```python
from build123d import *

# Parameters (mm, degrees)
SKETCH1_R               = 152.4
BOSS_EXTRUDE1_DEPTH     = 19.05
SKETCH5_R               = 55
CUT_EXTRUDE1_DEPTH      = 217.366407975
F_3_8_CLEARANCE_HOLE1_D = 9.8044


with BuildPart() as part:
    # Sketch1 → Boss-Extrude1 (new body)
    with BuildSketch(Plane.XY):
        with Locations(Location((0, 0, 0), (0, 0, 180))):
            Circle(SKETCH1_R)
    extrude(amount=BOSS_EXTRUDE1_DEPTH)

    # Sketch5 → Cut-Extrude1 (cut, through all)
    with BuildSketch(Plane(origin=(0, 0, 0), x_dir=(-1, 0, 0), z_dir=(0, 0, -1))):
        Circle(SKETCH5_R)
    extrude(amount=-CUT_EXTRUDE1_DEPTH, mode=Mode.SUBTRACT)

    # 3/8 Clearance Hole1 (through all)
    with Locations(Plane.XY.offset(19.05)):
        with Locations((60.285109168, 24.861699689), (60.262270723, -25.040419345), (-24.942124319, -60.287558469), (-60.212101884, -24.985282473), (24.959994735, -60.310396903), (-60.212101884, 24.861699689), (-24.88698742, 60.186814133), (25.015131626, 60.163975676)):
            Hole(F_3_8_CLEARANCE_HOLE1_D / 2)


solid = part.part
```
Geometry check sheet. Reference: the model listing, model coordinates, mm. Coordinates: 2 decimals unless noted, no trailing zeros. Order: outer loops, then holes, each group sorted by start corner. A loop starts at its lowest first (then second) coordinate and runs counter-clockwise, first axis right, second up.
Q1. Draft check along X on faces 1 (the face through (-27.2, -64.64, 9.39)), 2 (the face through (33.037, 148.776, 9.392)), 3 (the face through (-66, -2, 0)). Enter one of: released by +X, released by -X, zero draft, split by the parting line, or undercut.
Reply:
face 1: undercut
face 2: split by the parting line
face 3: zero draft
Q2. Sectioned sample at C-C on z = 6.75. Give the number of separate pieces and of enclosed holes in the cut face, and give its area (3 significant figures).
Reply:
separate pieces: 1
enclosed holes: 9
area: 62,900 mm2
Q3. Sectioned sample at A-A on x = 0. Record the cut outline in (y, z).
Reply:
outline: (-152.4, 0) - (-55, 0) - (-55, 19.05) - (-152.4, 19.05) - close; (55, 0) - (152.4, 0) - (152.4, 19.05) - (55, 19.05) - close
Q4. Depth check by flat-ended pin: pin 1 Ø1 at (y, z) = (-34.5, 6.5) entering from -X; pin 2 Ø5 at (y, z) = (68.5, 3.5) entering from -X; pin 3 Ø6 at (y, z) = (39, 6) entering from -X. Enter the tip coordinate at first touch or a pass-through.
Reply:
pin 1: stops at x = -148.56
pin 2: stops at x = -137.37
pin 3: stops at x = -148.09
Q5. Sectioned sample at D-D on y = -96.5. Record the cut outline in (x, z).
Reply:
outline: (-117.96, 0) - (117.96, 0) - (117.96, 19.05) - (-117.96, 19.05) - close
Q6. Thickness scan on probe 1 along Y at (x, z) = (-56.5, 8.75); probe 2 along X at (y, z) = (24.5, 15.25); probe 3 along X at (y, z) = (-56.5, 16.25). Record the ranges inside material, lowest first.
Reply:
probe 1: y = -141.54 to -28.19, -21.78 to 21.66, 28.06 to 141.54
probe 2: x = -150.42 to -65.1, -55.32 to -49.24, 49.24 to 55.4, 65.17 to 150.42
probe 3: x = -141.54 to -28.05, -21.83 to 21.88, 28.04 to 141.54
